Source: CAD feature listing. Evaluate the final solid. Frame: model axes, mm. A direction names the side the tool comes from. Give positions to 0.01 mm unless a question says otherwise; leave off trailing zeros. One line per question, with ' | ' between items. Start each with the question number.
(1) Pin query (flat end, axial travel): pin 1 (12 mm diameter, centred on x = 17.5, z = 26, fed in from -Y); pin 2 (1 mm diameter, centred on x = -65.5, y = -1.5, fed in from +Z); pin 3 (12 mm diameter, centred on y = 16, z = 19.5, fed in from +X). Return the tip coordinate at first contact, or that it passes through.
(2) Ray query, line 1 (Y direction, x = 0, z = 1); line 2 (X direction, y = -2.5, z = 7.5). Return the intervals inside material, ascending. Write a range as [from, to].
(3) Draft query along X for faces 3 (the cylindrical face through (12.758, -97.166, 3.112)), 4 (the cylindrical face through (-1.08, 54.88, 16.35)), 5 (the flat face through (52.2, -0.1, 0)). Return one class per face: +X half, -X half, draft (parallel to the pull), parting line (faces both ways), or undercut.
(4) Access query for faces 1 (the cylindrical face through (21.426, 16.429, 6.705)), 2 (the cylindrical face through (-55, 0, 16)). Directions: +Z, -Z, +X, -X, +Y, -Y. A direction counts if a zero-diameter tool reaches every point of the face in a straight line with its end or side. Return the directions, or none.
(5) Section A-A, the plane z = 26.5. State how many separate pieces and enclosed holes the cut face has, plus the area to 3 significant figures.
```python
from build123d import *

# Parameters (mm, degrees)
F2_R   = 5
F2_R_2 = 2


with BuildPart() as f1:
    # F0 (on Front) → F1 (revolve)
    with BuildSketch(Plane.XZ):
        with BuildLine():
            ThreePointArc((-92.8524549659, 15.3290077155), (-60.59962846, 33.9505314835), (-30.6264358238, 11.8459236323))
            ThreePointArc((-30.6264358238, 11.8459236323), (-30.1578548638, 10.1320014752), (-30, 8.3622051256))
            Line((-30, 8.3622051256), (-30, 5))
            Line((-30, 5), (-27.0000010729, 5))
            Line((-27.0000010729, 5), (-27.0000010729, 8.3622051256))
            ThreePointArc((-27.0000010729, 8.3622051256), (-27.2052123789, 10.6629401901), (-27.8143675765, 12.8910388105))
            ThreePointArc((-27.8143675765, 12.8910388105), (-60.4319668067, 36.9458416732), (-95.5303222531, 16.6814205056))
            ThreePointArc((-95.5303222531, 16.6814205056), (-97.3740624434, 11.6422043941), (-97.9999989271, 6.3129192238))
            Line((-97.9999989271, 6.3129192238), (-97.9999989271, 0))
            Line((-97.9999989271, 0), (-95, 0))
            Line((-95, 0), (-95, 6.3129192238))
            ThreePointArc((-95, 6.3129192238), (-94.4557073801, 10.9470804576), (-92.8524549659, 15.3290077155))
        make_face()
    revolve(axis=Axis((0, 0, 34.4163365662), (0, 0, 1)))

    # F2 (on face) → F3 (join, up to the next surface of F1)
    with BuildSketch(Plane(origin=(0, 0, 0), x_dir=(1, 0, 0), z_dir=(0, 0, -1))):
        with Locations((-50, 0)):
            Circle(F2_R)
        with Locations((-50, 0)):
            Circle(F2_R_2, mode=Mode.SUBTRACT)
        with Locations((0, -50)):
            Circle(F2_R)
        with Locations((0, -50)):
            Circle(F2_R_2, mode=Mode.SUBTRACT)
        with Locations((50, 0)):
            Circle(F2_R)
        with Locations((50, 0)):
            Circle(F2_R_2, mode=Mode.SUBTRACT)
        with Locations((0, 50)):
            Circle(F2_R)
        with Locations((0, 50)):
            Circle(F2_R_2, mode=Mode.SUBTRACT)
    extrude(until=Until.NEXT, dir=(0, 0, 1))


solid = f1.part
```
Check sheet entries:
1) pin 1: y = -92.13 | pin 2: z = 36.92 | pin 3: x = 95.72
2) line 1: [-98, -95], [-55, -52], [-48, -45], [45, 48], [52, 55], [95, 98] | line 2: [-97.94, -94.93], [-54.33, -45.67], [-29.9, -26.88], [26.88, 29.9], [45.67, 54.33], [94.93, 97.94]
3) face 3: parting line | face 4: undercut | face 5: draft
4) face 1: +Z, -Z | face 2: -Z
5) separate pieces: 6 | enclosed holes: 6 | area: 3,810 mm²
